Here's the drawing with two shaded views (mm, measured from the low corner). I have some questions. Coordinates: 2 decimals unless noted, no trailing zeros. Write each loop counter-clockwise with the first axis right and the second up, starting at its lowest first coordinate (ties: lowest second). Pieces come first, ordered by that corner, then holes.
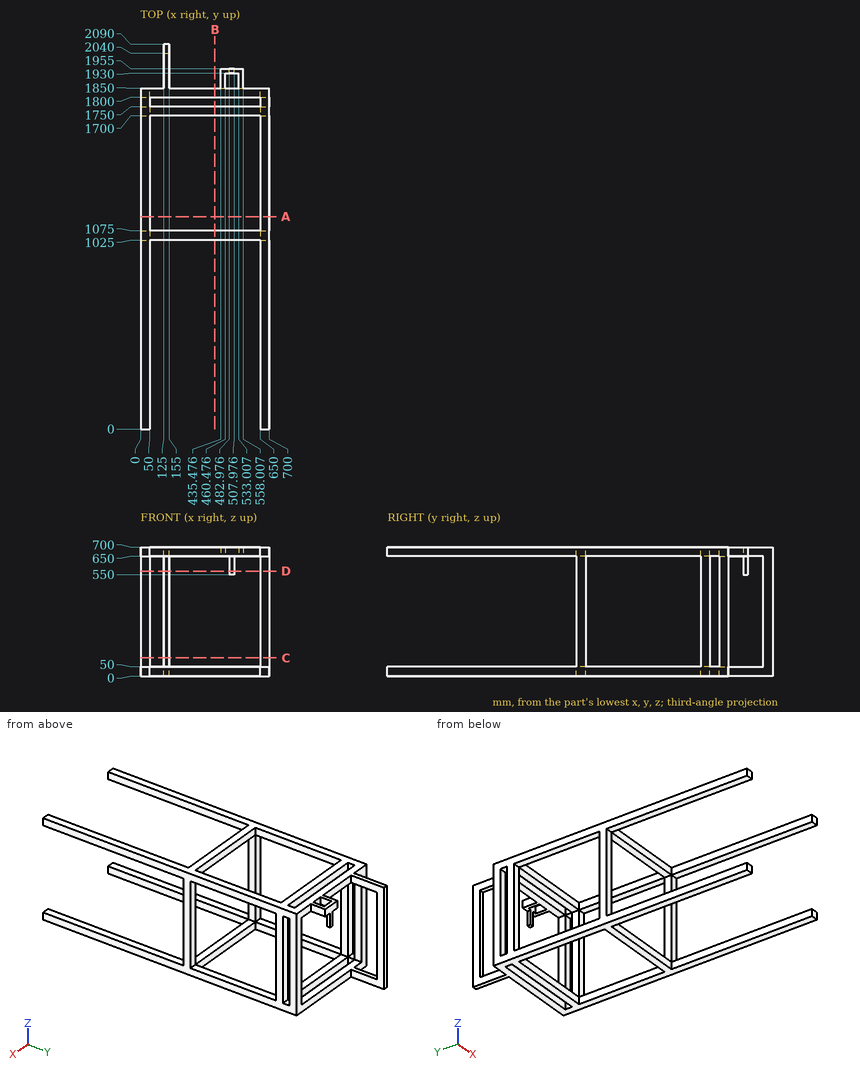
Item 1: If I drill on line 1 along Y through (x, z) = (663, 603); line 2 along Z through (x, y) = (653.5, 801.5); line 3 along X through (y, z) = (1854, 32), over which ranges is the centre line in solid material (lowest first)?
Item 2: Will these pins go through, and if not, where does the flat tip stop? pin 1 Ø7.5 at (x, y) = (489.5, 1941.5) entering from -Z; pin 2 Ø15 at (x, z) = (35, 299) entering from +Y.
Item 3: I want a section at B-B, the plane x = 404. List the corners of the cut face in (y, z) for me.
Item 4: I want a section at C-C, the plane z = 98.5. List the corners of the cut face in (x, y) for me.
Item 5: I want a section at D-D, the plane z = 569. Count the separate pieces of the cut face and the enclosed holes in it, then the cut area to 3 significant figures.
Item 6: I want a section at A-A, the plane y = 1153.5. List the corners of the cut face in (x, z) for me.
Taken from the geometry:
1. line 1: y = 1025 to 1075, 1700 to 1750, 1800 to 1850
1. line 2: z = 0 to 50, 650 to 700
1. line 3: x = 125 to 155
2. pin 1: stops at z = 550
2. pin 2: stops at y = 1850
3. outline: (1025, 0) - (1075, 0) - (1075, 50) - (1025, 50) - close; (1025, 650) - (1075, 650) - (1075, 700) - (1025, 700) - close; (1700, 0) - (1750, 0) - (1750, 50) - (1700, 50) - close; (1700, 650) - (1750, 650) - (1750, 700) - (1700, 700) - close; (1800, 0) - (1850, 0) - (1850, 50) - (1800, 50) - close; (1800, 650) - (1850, 650) - (1850, 700) - (1800, 700) - close
4. outline: (0, 1025) - (50, 1025) - (50, 1075) - (0, 1075) - close; (0, 1700) - (50, 1700) - (50, 1750) - (0, 1750) - close; (0, 1800) - (50, 1800) - (50, 1850) - (0, 1850) - close; (125, 2040) - (155, 2040) - (155, 2090) - (125, 2090) - close; (650, 1025) - (700, 1025) - (700, 1075) - (650, 1075) - close; (650, 1700) - (700, 1700) - (700, 1750) - (650, 1750) - close; (650, 1800) - (700, 1800) - (700, 1850) - (650, 1850) - close
5. separate pieces: 8
5. enclosed holes: 0
5. area: 17,100 mm2
6. outline: (0, 0) - (50, 0) - (50, 50) - (0, 50) - close; (0, 650) - (50, 650) - (50, 700) - (0, 700) - close; (650, 0) - (700, 0) - (700, 50) - (650, 50) - close; (650, 650) - (700, 650) - (700, 700) - (650, 700) - close
